from build123d import *

# Parameters (mm, degrees)
BOSS_EXTRUDE1_DEPTH = 13.9
SKETCH2_W           = 20
SKETCH2_H           = 11.5
BOSS_EXTRUDE2_DEPTH = 13.5
SKETCH4_W           = 24.8
SKETCH4_H           = 9.6
BOSS_EXTRUDE3_DEPTH = 3
BOSS_EXTRUDE4_START = -13.5
SKETCH5_W           = 22.5
SKETCH5_H           = 7.5
BOSS_EXTRUDE4_DEPTH = 13.5
CUT_EXTRUDE1_DEPTH  = 7
SKETCH7_R           = 1.75
CUT_EXTRUDE2_DEPTH  = 13.9


with BuildPart() as part:
    # Sketch1 → Boss-Extrude1 (new body)
    with BuildSketch(Plane.XY):
        with BuildLine():
            Line((0, 0), (20, 0))
            Line((20, 0), (20, 26.5))
            ThreePointArc((20, 26.5), (10, 36.5), (0, 26.5))
            Line((0, 26.5), (0, 0))
        make_face()
    extrude(amount=BOSS_EXTRUDE1_DEPTH)

    # Sketch2 → Boss-Extrude2 (add)
    with BuildSketch(Plane.XY.offset(13.9)):
        with Locations((10, 5.75)):
            Rectangle(SKETCH2_W, SKETCH2_H)
    extrude(amount=BOSS_EXTRUDE2_DEPTH)

    # Sketch4 → Boss-Extrude3 (add)
    with BuildSketch(Plane.XY.offset(13.9)):
        with Locations((10, 5.8)):
            Rectangle(SKETCH4_W, SKETCH4_H)
    extrude(amount=-BOSS_EXTRUDE3_DEPTH)

    # Sketch5 → Boss-Extrude4 (add)
    with BuildSketch(Plane.XY.offset(27.4).offset(BOSS_EXTRUDE4_START)):
        with Locations((10, 5.75)):
            Rectangle(SKETCH5_W, SKETCH5_H)
    extrude(amount=BOSS_EXTRUDE4_DEPTH)

    # Sketch6 → Cut-Extrude1 (cut)
    with BuildSketch(Plane.XY.offset(13.9)):
        Polygon((20, 11.5), (15.6, 11.5), (15.6, 10.75), (17.9, 10.75), (17.9, 9.5), (20, 9.5), align=None)
        Polygon((0, 0), (0, 2), (2.1, 2), (2.1, 0.75), (4.4, 0.75), (4.4, 0), align=None)
    extrude(amount=CUT_EXTRUDE1_DEPTH, mode=Mode.SUBTRACT)

    # Sketch7 → Cut-Extrude2 (cut)
    with BuildSketch(Plane(origin=(0, 0, 0), x_dir=(-1, 0, 0), z_dir=(0, 0, -1))):
        with Locations((-10, 26.5)):
            Circle(SKETCH7_R)
    extrude(amount=-CUT_EXTRUDE2_DEPTH, mode=Mode.SUBTRACT)


solid = part.part
Read the model definition and answer for the solid it produces. Units are mm, in the model's axes. A direction names the side the tool comes from. Round coordinates to 2 decimals unless told otherwise and drop trailing zeros. Order: outer loops, then holes, each group sorted by start corner. A loop starts at its lowest first (then second) coordinate and runs counter-clockwise, first axis right, second up.
1) Straight lines are drawn through the part: L1, parallel to Y at x = 10, z = 11; L2, parallel to Y at x = 21.25, z = 12.75; L3, parallel to X at y = 23.5, z = 11. For each, find the intervals that lie inside material, in ascending order.
2) The part is cut by section A-A on z = 14.75. Write down the section's boundary in (x, y).
3) The part is cut by section C-C on y = 2.5. Write down the section's boundary in (x, z).
4) Flat-ended cylindrical pins translate along their axes: pin 1 (1.9 mm diameter, centred on x = -1, y = 7.5, fed in from -Z); pin 2 (0.6 mm diameter, centred on x = 21, z = 20, fed in from -Y); pin 3 (0.6 mm diameter, centred on y = 1.5, z = 17.5, fed in from -X). Find the tip coordinate at first contact, or state that the pin passes through.
5) The mould has two halves that part along Z. Classify faces 1 (the face through (1.7, 0.8, 20.9)), 2 (the face through (10, 0, 14)), 3 (the face through (-1, 6, 10.9)), 4 (the face through (10, 6, 27.4)): released by +Z, released by -Z, zero draft, split by the parting line, or undercut.
6) For faces 5 (the face through (21.25, 6, 21)), 6 (the face through (21, 2, 21)), 7 (the face through (18, 11, 20.9)), 8 (the face through (-1, 9.5, 21)), determine the directions among +Z, -Z, +X, -X, +Y, -Y from which every point of the face is accessible in a straight line to the end or side of a thin tool.
7) The part is cut by section D-D on z = 9.25. Write down the section's boundary in (x, y).
8) The part is cut by section B-B on x = 10. Write down the section's boundary in (y, z), plus the area to 3 significant figures.
Resolved:
1. L1: y = 0 to 24.75, 28.25 to 36.5
1. L2: y = 1 to 10.6
1. L3: x = 0 to 20
2. outline: (-1.25, 2) - (2.1, 2) - (2.1, 0.75) - (4.4, 0.75) - (4.4, 0) - (20, 0) - (20, 2) - (21.25, 2) - (21.25, 9.5) - (17.9, 9.5) - (17.9, 10.75) - (15.6, 10.75) - (15.6, 11.5) - (0, 11.5) - (0, 9.5) - (-1.25, 9.5) - close
3. outline: (-2.4, 10.9) - (0, 10.9) - (0, 0) - (20, 0) - (20, 10.9) - (22.4, 10.9) - (22.4, 13.9) - (21.25, 13.9) - (21.25, 27.4) - (-1.25, 27.4) - (-1.25, 13.9) - (-2.4, 13.9) - close
4. pin 1: stops at z = 10.9
4. pin 2: stops at y = 2
4. pin 3: stops at x = 2.1
5. face 1: undercut
5. face 2: zero draft
5. face 3: released by -Z
5. face 4: released by +Z
6. face 5: +Z, +X, +Y, -Y
6. face 6: +Z, +X, -Y
6. face 7: +X, +Y
6. face 8: +Z, -X, +Y
7. outline: (0, 0) - (20, 0) - (20, 26.5) arc R10 ccw to (0, 26.5) - close; hole circle Ø3.5 at (10, 26.5)
8. outline: (0, 0) - (24.75, 0) - (24.75, 13.9) - (11.5, 13.9) - (11.5, 27.4) - (0, 27.4) - close; (28.25, 0) - (36.5, 0) - (36.5, 13.9) - (28.25, 13.9) - close
8. area: 614 mm2
